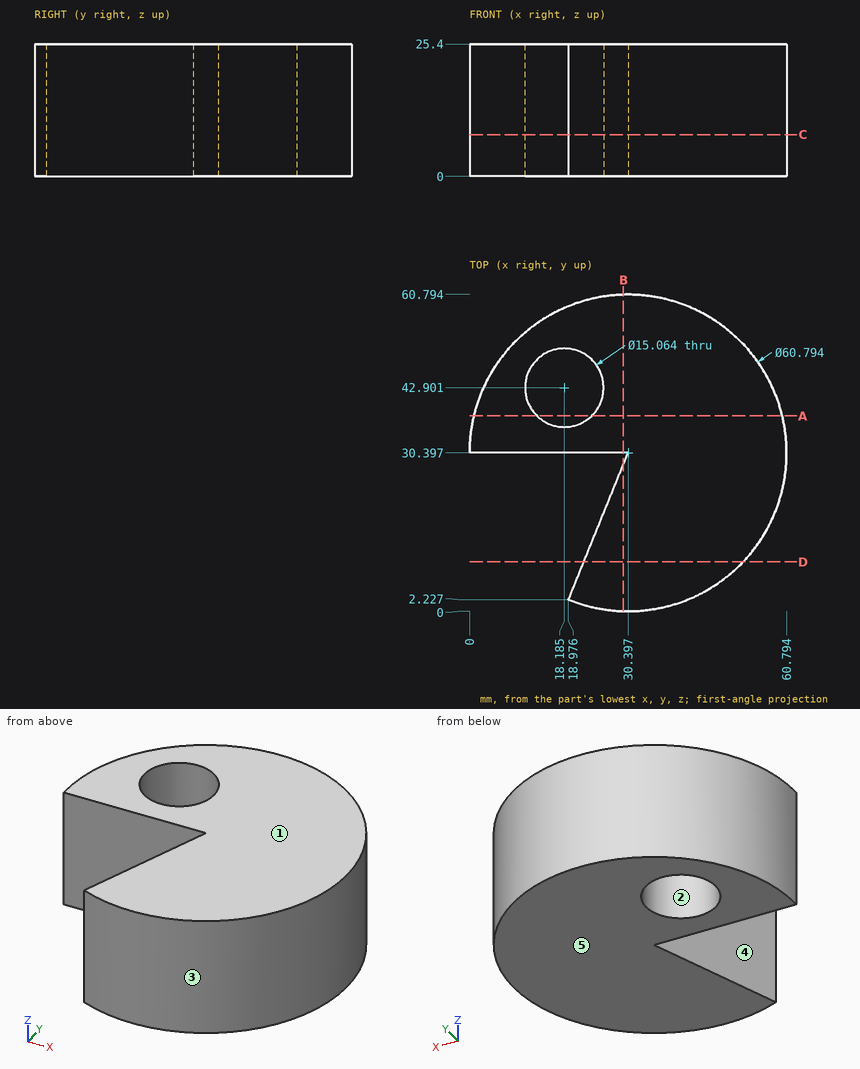
Geometry check sheet. Reference: drawing and pictorial views, mm from the part's lowest x, y, z. A direction names the side the tool comes from. Give positions to 0.01 mm unless a question says otherwise; leave off trailing zeros. Loops run counter-clockwise (first coordinate to the right, second up) from the corner with the lowest first, then second, coordinate; pieces in that order, holes last.
1. Mould release check, pull along X, two halves, no side actions. Record for the marked faces 1, 2 and 3: released by +X, released by -X, zero draft, split by the parting line, or undercut.
2. Set-up check for the marked faces 4 and 5: record each of +Z, -Z, +X, -X, +Y, -Y from which the full face is reachable in a straight line by a thin tool's end or side.
3. Go/stop test with flat-tipped pins: pin 1 Ø5 at (y, z) = (19, 11.5) entering from +X; pin 2 Ø12.5 at (x, z) = (20.5, 9) entering from -Y; pin 3 Ø6 at (y, z) = (14, 20.5) entering from +X; pin 4 Ø5 at (x, y) = (27, 34.5) entering from -Z. Record where each tip stops, or that it passes through.
4. Thickness scan on line 1 (X direction, y = 39, z = 3); line 2 (X direction, y = 36, z = 18.5) (1 decimal); line 3 (Y direction, x = 28.5, z = 10.75) (1 decimal). Record the ranges inside material, lowest first.
5. Section check D-D, the plane y = 9.5. Enter the section's corners in (x, z) (1 decimal), then the cut area to 3 significant figures.
6. Section check C-C, the plane z = 8. Enter the section's corners in (x, y) (1 decimal).
7. Section check A-A, the plane y = 37.5. Enter the section's corners in (x, z) (1 decimal).
8. Section check B-B, the plane x = 29.5. Enter the section's corners in (y, z) (1 decimal).
Geometry says:
1. face 1: zero draft
1. face 2: undercut
1. face 3: split by the parting line
2. face 4: +Z, -Z, -X
2. face 5: -Z, +X, -X, +Y, -Y
3. pin 1: stops at x = 59.46
3. pin 2: stops at y = 0.22
3. pin 3: stops at x = 57.68
3. pin 4: stops at z = 0
4. line 1: x = 1.24 to 11.74, 24.63 to 59.55
4. line 2: x = 0.5 to 15.2, 21.2 to 60.3
4. line 3: y = 0.1 to 25.7, 30.4 to 60.7
5. outline: (21.9, 0) - (52.5, 0) - (52.5, 25.4) - (21.9, 25.4) - close
5. area: 776 mm2
6. outline: (0, 30.4) - (30.4, 30.4) - (19, 2.2) arc R30.4 ccw (long way) to start; hole circle Ø15.1 at (18.2, 42.9)
7. outline: (0.8, 0) - (12.9, 0) - (12.9, 25.4) - (0.8, 25.4) - close; (23.4, 0) - (60, 0) - (60, 25.4) - (23.4, 25.4) - close
8. outline: (0, 0) - (28.2, 0) - (28.2, 25.4) - (0, 25.4) - close; (30.4, 0) - (60.8, 0) - (60.8, 25.4) - (30.4, 25.4) - close
